Read the model definition and answer for the solid it produces. Units are mm, in the model's axes. Face numbers are marked on the shaded views. Give positions to 0.01 mm unless a question says otherwise; leave off trailing zeros. Write each loop counter-clockwise with the first axis right and the second up, starting at its lowest first coordinate (ties: lowest second). Pieces come first, ordered by that corner, then holes. Notation, with made-up numbers: (0.5, -11) -> (14.5, -11) arc R27 ccw to (14.5, 10) -> close; hole circle Ø4 at (27, 11). An arc over 180 degrees is marked (long way). Answer as CSV lines item,"result". Start each with the question number.
1. For a pull along Y with two mould halves and no side action, classify the marked faces 1 and 2 as pulls with the +Y half, pulls with the -Y half, needs draft (parallel to the pull), parting line crosses it, or undercut.
2. The part is cut by section C-C, the plane x = 1.5. Determine the outline of the cut face in (y, z) (3 decimals).
3. The part is cut by section B-B, the plane x = 33. Determine the outline of the cut face in (y, z) (3 decimals), and give its area (3 significant figures).
4. The part is cut by section A-A, the plane x = -31.75. Determine the outline of the cut face in (y, z) (3 decimals).
5. Given pin 1 (1 mm diameter, centred on y = -0.5, z = 2, fed in from +X); pin 2 (1.7 mm diameter, centred on y = -1.5, z = 2.5, fed in from -X); pin 3 (6 mm diameter, centred on x = -31.75, y = 12.7, fed in from +Z), each flat-ended and moving along its own axis, determine where each tip first touches the part or whether it passes through.
6. Find the intervals of material crossed by line 1 (Y direction, x = -5.5, z = 3.25); line 2 (Y direction, x = -31.75, z = 3.85) (3 decimals); line 3 (Y direction, x = 29.5, z = 2.5) (3 decimals), in increasing order.
7. The part is cut by section D-D, the plane z = 2. Give the number of separate pieces and of enclosed holes in the cut face, and give its area (3 significant figures).
from build123d import *

# Parameters (mm, degrees)
SKETCH1_W           = 50.8
SKETCH1_H           = 76.2
BOSS_EXTRUDE1_DEPTH = 6.477
SKETCH3_W           = 76.2
SKETCH3_H           = 13.97
CUT_EXTRUDE2_DEPTH  = 3.048
SKETCH2_R           = 2.38125
SKETCH2_W           = 12.7
SKETCH2_H           = 13.97
SKETCH2_W_2         = 21.082
CUT_EXTRUDE1_DEPTH  = 47.24631368
FILLET1_R           = 3.302
SKETCH5_W           = 23.876
SKETCH5_H           = 3.302
CUT_EXTRUDE3_DEPTH  = 47.24631368
SKETCH6_W           = 23.876
SKETCH6_H           = 1.016
CUT_EXTRUDE4_DEPTH  = 3.302
FILLET4_R           = 1.5875
FILLET5_R           = 1.5875
CHAMFER1_SIZE       = 1.27


with BuildPart() as part:
    # Sketch1 → Boss-Extrude1 (new body)
    with BuildSketch(Plane(origin=(0, 0, 0), x_dir=(0, 1, 0), z_dir=(0, 0, 1))):
        Rectangle(SKETCH1_W, SKETCH1_H)
    extrude(amount=BOSS_EXTRUDE1_DEPTH)

    # Sketch3 → Cut-Extrude2 (cut)
    with BuildSketch(Plane.XY.offset(6.477)):
        Rectangle(SKETCH3_W, SKETCH3_H)
    extrude(amount=-CUT_EXTRUDE2_DEPTH, mode=Mode.SUBTRACT)

    # Sketch2 → Cut-Extrude1 (cut, through all)
    with BuildSketch(Plane.XY.offset(6.477)):
        with Locations((-31.75, 12.7)):
            Circle(SKETCH2_R)
        with Locations((-31.75, -12.7)):
            Circle(SKETCH2_R)
        with Locations((-31.75, 0)):
            Rectangle(SKETCH2_W, SKETCH2_H)
        with Locations((27.559, 0)):
            Rectangle(SKETCH2_W_2, SKETCH2_H)
    extrude(amount=-CUT_EXTRUDE1_DEPTH, mode=Mode.SUBTRACT)

    # Fillet1
    fillet1_edges = [part.edges().sort_by_distance(p)[0] for p in [
        (-25.4, 6.985, 1.7145),
        (-25.4, -6.985, 1.7145),
        (17.018, 6.985, 1.7145),
        (17.018, -6.985, 1.7145),
    ]]
    fillet(fillet1_edges, radius=FILLET1_R)

    # Sketch5 → Cut-Extrude3 (cut, through all)
    with BuildSketch(Plane.XY.offset(6.477)):
        with Locations((0, 12.7)):
            Rectangle(SKETCH5_W, SKETCH5_H)
    cut_extrude3 = extrude(amount=-CUT_EXTRUDE3_DEPTH, mode=Mode.SUBTRACT)

    # Sketch6 → Cut-Extrude4 (cut)
    with BuildSketch(Plane.XY.offset(6.477)):
        with Locations((0, 10.541)):
            Rectangle(SKETCH6_W, SKETCH6_H)
    cut_extrude4 = extrude(amount=-CUT_EXTRUDE4_DEPTH, mode=Mode.SUBTRACT)

    # Mirror1: Cut-Extrude3, Cut-Extrude4 across plane
    add(cut_extrude3.mirror(Plane.ZX), mode=Mode.SUBTRACT)
    add(cut_extrude4.mirror(Plane.ZX), mode=Mode.SUBTRACT)

    # Fillet4
    fillet4_edges = [part.edges().sort_by_distance(p)[0] for p in [
        (11.938, 14.351, 3.2385),
        (11.938, 11.049, 1.5875),
        (-11.938, 11.049, 1.5875),
        (-11.938, 14.351, 3.2385),
        (11.938, -11.049, 1.5875),
        (11.938, -14.351, 3.2385),
        (-11.938, -14.351, 3.2385),
        (-11.938, -11.049, 1.5875),
    ]]
    fillet(fillet4_edges, radius=FILLET4_R)

    # Fillet5
    fillet5_edges = [part.edges().sort_by_distance(p)[0] for p in [
        (-11.938, 10.033, 4.826),
        (11.938, 10.033, 4.826),
        (-11.938, -10.033, 4.826),
        (11.938, -10.033, 4.826),
    ]]
    fillet(fillet5_edges, radius=FILLET5_R)

    # Chamfer1
    chamfer1_edges = [part.edges().sort_by_distance(p)[0] for p in [
        (-34.13125, 12.7, 6.477),
        (-34.13125, -12.7, 6.477),
    ]]
    chamfer(chamfer1_edges, length=CHAMFER1_SIZE)


solid = part.part
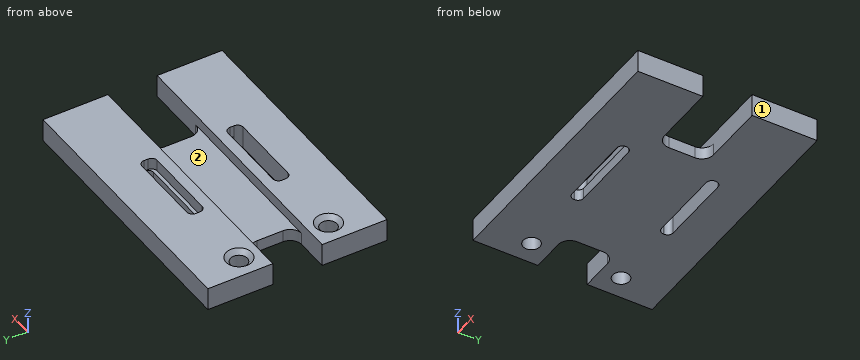
Results found:
1,face 1,"needs draft"
1,face 2,"undercut"
2,outline,"(-25.4, 0) -> (-14.351, 0) -> (-14.351, 6.477) -> (-25.4, 6.477) -> close; (-11.049, 0) -> (11.049, 0) -> (11.049, 3.175) -> (10.033, 3.175) -> (10.033, 6.477) -> (6.985, 6.477) -> (6.985, 3.429) -> (-6.985, 3.429) -> (-6.985, 6.477) -> (-10.033, 6.477) -> (-10.033, 3.175) -> (-11.049, 3.175) -> close; (14.351, 0) -> (25.4, 0) -> (25.4, 6.477) -> (14.351, 6.477) -> close"
3,outline,"(-25.4, 0) -> (-6.985, 0) -> (-6.985, 6.477) -> (-25.4, 6.477) -> close; (6.985, 0) -> (25.4, 0) -> (25.4, 6.477) -> (6.985, 6.477) -> close"
3,area,"239 mm²"
4,outline,"(-25.4, 0) -> (-15.081, 0) -> (-15.081, 5.207) -> (-16.351, 6.477) -> (-25.4, 6.477) -> close; (-10.319, 0) -> (-6.985, 0) -> (-6.985, 6.477) -> (-9.049, 6.477) -> (-10.319, 5.207) -> close; (6.985, 0) -> (10.319, 0) -> (10.319, 5.207) -> (9.049, 6.477) -> (6.985, 6.477) -> close; (15.081, 0) -> (25.4, 0) -> (25.4, 6.477) -> (16.351, 6.477) -> (15.081, 5.207) -> close"
5,pin 1,"stops at x = 17.02"
5,pin 2,"stops at x = -25.4"
5,pin 3,"stops at z = 5.83"
6,line 1,"y = -25.4 to -14.35, -10.03 to 10.03, 14.35 to 25.4"
6,line 2,"y = -25.4 to -15.081, -10.319 to -6.985, 6.985 to 10.319, 15.081 to 25.4"
6,line 3,"y = -25.4 to -6.985, 6.985 to 25.4"
7,separate pieces,"1"
7,enclosed holes,"4"
7,area,"3,220 mm²"
